Autodesk Inventor part; units mm, degrees
ref_plane "YZ Plane" through (0, 0, 0) normal (1, 0, 0) x (0, 1, 0)
ref_plane "XZ Plane" through (0, 0, 0) normal (0, 1, 0) x (-1, 0, 0)
ref_plane "XY Plane" through (0, 0, 0) normal (0, 0, 1) x (1, 0, 0)
sketch "Sketch1" plane through (0, 0, 0) normal (0, 0, 1) x (1, 0, 0)
  line L0 (279.4, 0) -> (279.4, 304.8)
  line L1 (279.4, 304.8) -> (0, 304.8)
  line L2 (0, 304.8) -> (0, 0)
  line L3 (31.75, 0) -> (31.75, 266.7)
  line L4 (31.75, 266.7) -> (247.65, 266.7)
  line L5 (247.65, 266.7) -> (247.65, 0)
  line L6 (247.65, 0) -> (279.4, 0)
  line L7 (31.75, 0) -> (0, 0)
  point P0 (139.7, 152.4)
  point P1 (139.7, 289.941)
  point P2 (20.586, 221.1705)
  point P3 (20.586, 83.6295)
  point P4 (139.7, 14.859)
  point P5 (258.814, 83.6295)
  point P6 (258.814, 221.1705)
  dimension "d0" = 279.4
  dimension "d1" = 304.8
  dimension "d2" = 139.7
  dimension "d3" = 152.4
  dimension "d4" = 137.541
  dimension "d7" = 360
  dimension "d9" = 31.75
  dimension "d10" = 31.75
  dimension "d11" = 38.1
extrude "Extrusion1" add sketch "Sketch1" against normal blind 3.175
hole "Hole1" at (139.7, 152.4, 0) at (139.7, 289.941, 0) at (20.586, 221.1705, 0) at (20.586, 83.6295, 0) at (139.7, 14.859, 0) at (258.814, 83.6295, 0) at (258.814, 221.1705, 0) direction (0, 0, -1) diameter 6.35 depth 25.4 tip angle 118
properties part number "middle-top spacer plate"
Verification items for the finished model (mm, model axes). Coordinates: 2 decimals unless noted, no trailing zeros. Order: outer loops, then holes, each group sorted by start corner. A loop starts at its lowest first (then second) coordinate and runs counter-clockwise, first axis right, second up. Notation, with made-up numbers: M -1.5,17.5 L 53.5,17.5 A30 cw 53.5,45.5 Z; hole C 19.25,-18 d9. An arc over 180 degrees is marked long. One line per item, written item: value. Start each with the question number.
Item 1: Mould release check, pull along Y, two halves, no side actions. Record for faces 1 (the flat face through (118, 277, -3.175)), 2 (the cylindrical face through (19.63, 80.6, -1.61)): pulls with the +Y half, pulls with the -Y half, needs draft (parallel to the pull), parting line crosses it, or undercut.
Item 2: Depth check by flat-ended pin: P1, Ø1, axis at x = 171.5, z = -1.5, coming from the -Y side. Enter the tip coordinate at first touch or a pass-through.
Item 3: Sectioned sample at A-A on y = 64. Record the cut outline in (x, z) (3 decimals).
Item 4: Sectioned sample at B-B on z = -1.9. Give the number of separate pieces and of enclosed holes in the cut face, then the cut area to 3 significant figures.
Item 5: Thickness scan on probe 1 along X at (y, z) = (35, -0.3); probe 2 along Y at (x, z) = (260, -2.75); probe 3 along Y at (x, z) = (23.5, -0.25). Record the ranges inside material, lowest first.
Item 6: Sectioned sample at C-C on x = 162. Record the cut outline in (y, z) (3 decimals), then the cut area to 3 significant figures.
Calculated:
1. face 1: needs draft
1. face 2: undercut
2. P1: y = 266.7
3. outline: M 0,-3.175 L 31.75,-3.175 L 31.75,0 L 0,0 Z; M 247.65,-3.175 L 279.4,-3.175 L 279.4,0 L 247.65,0 Z
4. separate pieces: 1
4. enclosed holes: 5
4. area: 27,400 mm^2
5. probe 1: 0 to 31.75, 247.65 to 279.4
5. probe 2: 0 to 80.68, 86.57 to 218.23, 224.12 to 304.8
5. probe 3: 0 to 82.37, 84.89 to 219.91, 222.43 to 304.8
6. outline: M 266.7,-3.175 L 304.8,-3.175 L 304.8,0 L 266.7,0 Z
6. area: 121 mm^2
